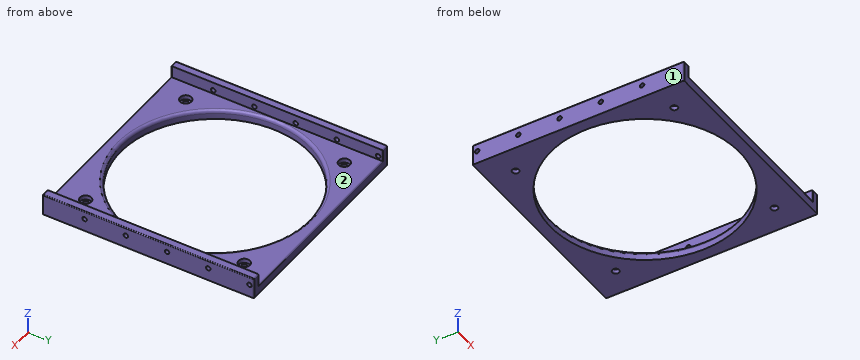
from build123d import *

# Parameters (mm, degrees)
SKETCH003_W          = 140
SKETCH003_H          = 140
SKETCH003_R          = 2.25
SKETCH003_R_2        = 62.5
PAD_DEPTH            = 6
SKETCH009_W          = 5
SKETCH009_H          = 140
PAD003_DEPTH         = 8
SKETCH010_R          = 3.75
POCKET002_DEPTH      = 3
SKETCH011_R          = 1.5
POCKET003_DEPTH      = 70.001
POCKET003_DEPTH_BACK = 70.001
LINEARPATTERN_COUNT  = 5
LINEARPATTERN_PITCH  = 27.3
FILLET_R             = 2
FILLET001_R          = 0.6


with BuildPart() as part:
    # Sketch003 → Pad (new body)
    with BuildSketch(Plane.XY):
        Rectangle(SKETCH003_W, SKETCH003_H)
        with Locations((52.5, 52.5)):
            Circle(SKETCH003_R, mode=Mode.SUBTRACT)
        with Locations((52.5, -52.5)):
            Circle(SKETCH003_R, mode=Mode.SUBTRACT)
        with Locations((-52.5, -52.5)):
            Circle(SKETCH003_R, mode=Mode.SUBTRACT)
        with Locations((-52.5, 52.5)):
            Circle(SKETCH003_R, mode=Mode.SUBTRACT)
        Circle(SKETCH003_R_2, mode=Mode.SUBTRACT)
    extrude(amount=PAD_DEPTH)

    # Sketch009 → Pad003 (join)
    with BuildSketch(Plane.XY.offset(6)):
        with Locations((-67.5, 0)):
            Rectangle(SKETCH009_W, SKETCH009_H)
        with Locations((67.5, 0)):
            Rectangle(SKETCH009_W, SKETCH009_H)
    extrude(amount=PAD003_DEPTH)

    # Sketch010 → Pocket002 (cut)
    with BuildSketch(Plane.XY.offset(6)):
        with Locations((52.5, 52.5)):
            Circle(SKETCH010_R)
        with Locations((-52.5, 52.5)):
            Circle(SKETCH010_R)
        with Locations((-52.5, -52.5)):
            Circle(SKETCH010_R)
        with Locations((52.5, -52.5)):
            Circle(SKETCH010_R)
    extrude(amount=-POCKET002_DEPTH, mode=Mode.SUBTRACT)

    # Sketch011 → Pocket003 (cut, two sides)
    with BuildSketch(Plane.YZ) as pocket003_sk:
        with Locations((67, 8.5)):
            Circle(SKETCH011_R)
    pocket003 = extrude(amount=-POCKET003_DEPTH, mode=Mode.SUBTRACT) + extrude(pocket003_sk.sketch, amount=POCKET003_DEPTH_BACK, mode=Mode.SUBTRACT)

    # LinearPattern: Pocket003 ×5
    with Locations(*[(0, -i * LINEARPATTERN_PITCH, 0) for i in range(1, LINEARPATTERN_COUNT)]):
        add(pocket003, mode=Mode.SUBTRACT)

    # Fillet
    fillet_edges = [part.edges().sort_by_distance(p)[0] for p in [
        (-62.5, 0, 6),
    ]]
    fillet(fillet_edges, radius=FILLET_R)

    # Fillet001
    fillet001_edges = [part.edges().sort_by_distance(p)[0] for p in [
        (67.5, -70, 14),
        (70, -70, 7),
        (70, 0, 14),
        (67.5, 70, 14),
        (70, 70, 7),
        (0, 70, 6),
        (0, -70, 6),
        (-67.5, -70, 14),
        (-70, -70, 7),
        (-70, 0, 14),
        (-67.5, 70, 14),
        (-70, 70, 7),
        (-65, 70, 10),
        (-65, -70, 10),
        (65, -70, 10),
        (65, 70, 10),
    ]]
    fillet(fillet001_edges, radius=FILLET001_R)


solid = part.part
Here's how the part is built. I have some questions about the finished solid (model axes, mm). Face numbers are marked on the shaded views. A direction names the side the tool comes from. Coordinates: 2 decimals unless noted, no trailing zeros. Write each loop counter-clockwise with the first axis right and the second up, starting at its lowest first coordinate (ties: lowest second). Pieces come first, ordered by that corner, then holes.
Item 1: If I drill on line 1 (X direction, y = -57.5, z = 11.25); line 2 (Z direction, x = 67.4, y = -14.9); line 3 (Y direction, x = 52.5, z = 0.75), over which ranges is the centre line in solid material (lowest first)?
Item 2: On a 3-axis mill with a long thin cutter (end or side, diameter ignored), from which of +Z, -Z, +X, -X, +Y, -Y can I reach the whole of each face in a straight line? I mean the marked faces 1 and 2. Say none if no direction works.
Item 3: Will these pins go through, and if not, where does the flat tip stop? pin 1 (10 mm diameter, centred on x = 52.5, y = 52.5, fed in from -Z); pin 2 (5 mm diameter, centred on x = 51, y = 34.5, fed in from +Z); pin 3 (2 mm diameter, centred on x = -54, y = 50.5, fed in from +Z); pin 4 (1.8 mm diameter, centred on y = 39.7, z = 8.5, fed in from -X).
Item 4: I want a section at C-C on x = -52.5. Count the separate pieces of the cut face and the enclosed holes in it, and give its area (3 significant figures).
Item 5: I want a section at A-A on y = 0. Write out the boundary of the cut face in (x, z), and give its area (3 significant figures).
Item 6: I want a section at B-B on x = 0. Write out the boundary of the cut face in (y, z).
Findings below:
1. line 1: x = -70 to -65, 65 to 70
1. line 2: z = 0 to 7, 10 to 14
1. line 3: y = -70 to -54.75, -50.25 to -33.91, 33.91 to 50.25, 54.75 to 70
2. face 1: +Z, -Z, -X, +Y, -Y
2. face 2: +Z, +Y, -Y
3. pin 1: stops at z = 0
3. pin 2: stops at z = 5.95
3. pin 3: stops at z = 3
3. pin 4: passes through
4. separate pieces: 4
4. enclosed holes: 0
4. area: 358 mm2
5. outline: (-70, 0) - (-62.5, 0) - (-62.5, 4) arc R2 ccw to (-64.5, 6) - (-65, 6) - (-65, 14) - (-69.4, 14) arc R0.6 ccw to (-70, 13.4) - close; (62.5, 0) - (70, 0) - (70, 13.4) arc R0.6 ccw to (69.4, 14) - (65, 14) - (65, 6) - (64.5, 6) arc R2 ccw to (62.5, 4) - close
5. area: 168 mm2
6. outline: (-70, 0) - (-62.5, 0) - (-62.5, 4) arc R2 ccw to (-64.5, 6) - (-69.4, 6) arc R0.6 ccw to (-70, 5.4) - close; (62.5, 0) - (70, 0) - (70, 5.4) arc R0.6 ccw to (69.4, 6) - (64.5, 6) arc R2 ccw to (62.5, 4) - close
